Design review of the part built by this model. Coordinates are the model's own, in mm. A direction names the side the tool comes from. Give positions to 0.01 mm unless a question says otherwise; leave off trailing zeros. Write each loop counter-clockwise with the first axis right and the second up, starting at its lowest first coordinate (ties: lowest second). Pieces come first, ordered by that corner, then holes. Notation, with made-up numbers: (-30, 21.25) -> (-18, 21.25) arc R12 ccw to (-18, 29.25) -> close; hole circle Ø7 at (30.5, 39.25). An arc over 180 degrees is marked (long way). Answer as a JSON object with one key per item and string values.
Autodesk Inventor part; units mm, degrees
ref_plane "YZ Plane" through (0, 0, 0) normal (1, 0, 0) x (0, 1, 0)
ref_plane "XZ Plane" through (0, 0, 0) normal (0, 1, 0) x (-1, 0, 0)
ref_plane "XY Plane" through (0, 0, 0) normal (0, 0, 1) x (1, 0, 0)
sketch "Sketch1" plane through (0, 0, 0) normal (0, 0, 1) x (1, 0, 0)
  line L0 (0, 0) -> (50.8, 0)
  line L1 (50.8, 0) -> (50.8, 38.1)
  line L2 (0, 38.1) -> (0, 0)
  line L3 (3.175, 38.1) -> (3.175, 3.175)
  line L4 (3.175, 3.175) -> (47.625, 3.175)
  line L5 (47.625, 3.175) -> (47.625, 38.1)
  line L6 (50.8, 38.1) -> (47.625, 38.1)
  line L7 (3.175, 38.1) -> (0, 38.1)
  dimension "d0" = 38.1
  dimension "d1" = 50.8
  dimension "d2" = 3.175
  dimension "d3" = 3.175
  dimension "d4" = 3.175
extrude "Extrusion1" add sketch "Sketch1" along normal blind 25.4
sketch "Sketch2" plane through (50.8, 0, 0) normal (1, 0, 0) x (0, 0, -1)
  line L0 (-25.4, 38.1) -> (-25.4, 0)
  line L1 (0, 0) -> (-25.4, 0)
  line L2 (0, 0) -> (0, 38.1)
  line L3 (0, 38.1) -> (-25.4, 38.1)
  circle A0 centre (-7.9375, 30.1625) radius 4.7625
  arc A1 (0, 30.1625) -> (-15.532, 32.4705) centre (-7.9375, 30.1625) ccw
  line L4 (-25.4, 0) -> (-15.532, 32.4705)
  line L5 (0, 30.1625) -> (0, 0)
  dimension "d7" = 9.525
  dimension "d8" = 30.1625
  dimension "d9" = 17.4625
extrude "Extrusion2" cut sketch "Sketch2" against normal through all contours L3 A1 L4 L0 | L3 L2 A1 | A0
sketch "Sketch3" plane through (0, 0, 25.4) normal (0, -1, 0) x (1, 0, 0)
  line L0 (0, -25.4) -> (0, 0)
  line L1 (0, -25.4) -> (50.8, -25.4)
  line L2 (50.8, -25.4) -> (50.8, 0)
  circle A0 centre (12.7, -12.7) radius 3.175
  circle A1 centre (38.1, -12.7) radius 3.175
  dimension "d12" = 6.35
  dimension "d13" = 6.35
  dimension "d14" = 12.7
  dimension "d15" = 12.7
  dimension "d16" = 12.7
extrude "Extrusion3" cut sketch "Sketch3" against normal through all
equation "\"d3\" = d2"
equation "\"d4\" = d3"
equation "\"d13\" = d12"
equation "\"d15\" = d14"
equation "\"d16\" = d15"
properties part number "manipulator U bracket"
(1) For line 1 along X through (y, z) = (7.5, 6.75) (3 decimals); line 2 along Y through (x, z) = (15.5, 3.25) (3 decimals); line 3 along Z through (x, y) = (38, 2), list the stretches that pass through material, from the lowest coordinate up.
Here are the results:
{"line 1": "x = 0 to 3.175, 47.625 to 50.8", "line 2": "y = 0 to 3.175", "line 3": "z = 0 to 9.53, 15.87 to 24.79"}
(2) Clearance check with a flat-ended pin moving along its axis: pin 1 (7.5 mm diameter, centred on x = 12.7, z = 12.7, fed in from +Y) (3 decimals). State where the tip first meets the part, or that it passes through.
Here are the results:
{"pin 1": "stops at y = 3.175"}
(3) We need section B-B, the plane y = 29. State the section outline as (x, z) points (3 decimals).
Here are the results:
{"outline": "(0, 0) -> (3.175, 0) -> (3.175, 3.319) -> (0, 3.319) -> close; (0, 12.556) -> (3.175, 12.556) -> (3.175, 16.587) -> (0, 16.587) -> close; (47.625, 0) -> (50.8, 0) -> (50.8, 3.319) -> (47.625, 3.319) -> close; (47.625, 12.556) -> (50.8, 12.556) -> (50.8, 16.587) -> (47.625, 16.587) -> close"}
(4) We need section D-D, the plane y = 16. State the section outline as (x, z) points (1 decimal).
Here are the results:
{"outline": "(0, 0) -> (3.2, 0) -> (3.2, 20.5) -> (0, 20.5) -> close; (47.6, 0) -> (50.8, 0) -> (50.8, 20.5) -> (47.6, 20.5) -> close"}
(5) We need section A-A, the plane x = 38.1. State the section outline as (y, z) points (3 decimals), then the cut area to 3 significant figures.
Here are the results:
{"outline": "(0, 0) -> (3.175, 0) -> (3.175, 9.525) -> (0, 9.525) -> close; (0, 15.875) -> (3.175, 15.875) -> (3.175, 24.435) -> (0, 25.4) -> close", "area": "59.0 mm²"}
(6) The part is to be moulded in two halves that separate along Z. For faces 1 (the cylindrical face through (34.93, 1.57, 12.84)), 2 (the flat face through (25, 0, 13)), 3 (the flat face through (25.52, 2.93, 24.51)), 4 (the cylindrical face through (10.18, 1.57, 10.77)), say which applies: +Z half, -Z half, draft (parallel to the pull), parting line (faces both ways), or undercut.
Here are the results:
{"face 1": "undercut", "face 2": "draft", "face 3": "+Z half", "face 4": "undercut"}
(7) We need section C-C, the plane z = 12. State the section outline as (x, y) points (3 decimals), then the cut area to 3 significant figures.
Here are the results:
{"outline": "(0, 0) -> (9.603, 0) -> (9.603, 3.175) -> (3.175, 3.175) -> (3.175, 27.677) -> (0, 27.677) -> close; (0, 32.648) -> (3.175, 32.648) -> (3.175, 36.982) -> (0, 36.982) -> close; (15.797, 0) -> (35.003, 0) -> (35.003, 3.175) -> (15.797, 3.175) -> close; (41.197, 0) -> (50.8, 0) -> (50.8, 27.677) -> (47.625, 27.677) -> (47.625, 3.175) -> (41.197, 3.175) -> close; (47.625, 32.648) -> (50.8, 32.648) -> (50.8, 36.982) -> (47.625, 36.982) -> close", "area": "305 mm²"}
(8) For faces 5 (the flat face through (0, 15, 10)), 6 (the flat face through (25, 3.175, 12)), list the 3-axis set-ups (+Z, -Z, +X, -X, +Y, -Y) from which the entire face can be reached by the end or side of a thin tool; tool diameter is ignored.
Here are the results:
{"face 5": "+Z, -Z, -X, +Y, -Y", "face 6": "+Z, -Z, +Y"}
